Check sheet for the modelled part. Datum: model origin and axes. Units: mm. A direction names the side the tool comes from. Give positions to 0.01 mm unless a question says otherwise; leave off trailing zeros. Order: outer loops, then holes, each group sorted by start corner. A loop starts at its lowest first (then second) coordinate and runs counter-clockwise, first axis right, second up. Notation, with made-up numbers: M 83.25,67.25 L 134.25,67.25 A24 cw 134.25,99.25 Z; hole C 40.25,83.5 d9. An arc over 180 degrees is marked long. Answer in a Markdown table with one row per item. Add a question column.
Autodesk Inventor part; units mm, degrees
ref_plane "YZ Plane" through (0, 0, 0) normal (1, 0, 0) x (0, 1, 0)
ref_plane "XZ Plane" through (0, 0, 0) normal (0, 1, 0) x (-1, 0, 0)
ref_plane "XY Plane" through (0, 0, 0) normal (0, 0, 1) x (1, 0, 0)
sketch "Sketch1" plane through (0, 0, 0) normal (0, 1, 0) x (-1, 0, 0)
  line L0 (0, 0) -> (-120.65, 0)
  line L1 (-120.65, 0) -> (-120.65, -63.5)
  line L2 (-120.65, -63.5) -> (0, -63.5)
  line L3 (0, -63.5) -> (0, 0)
  dimension "d0" = 120.65
  dimension "d1" = 63.5
extrude "Extrusion1" add sketch "Sketch1" along normal blind 3.175
sketch "Sketch2" plane through (0, 0, 0) normal (0, 0, 1) x (1, 0, 0)
  line L0 (0, 0) -> (120.65, 0)
  line L1 (0, 0) -> (120.65, 0)
  line L2 (120.65, 0) -> (120.65, -31.75)
  line L3 (120.65, -31.75) -> (0, -31.75)
  line L4 (0, -31.75) -> (0, 0)
  dimension "d4" = 31.75
extrude "Extrusion2" add sketch "Sketch2" against normal blind 3.175
sketch "Sketch4" plane through (120.65, 0, -63.5) normal (0, 0, -1) x (-1, 0, 0)
  line L0 (0, -31.75) -> (0, 3.175)
  line L1 (120.65, -31.75) -> (120.65, 3.175)
  line L2 (0, 3.175) -> (120.65, 3.175)
  line L3 (120.65, 3.175) -> (120.65, -31.75)
  line L4 (120.65, -31.75) -> (0, -31.75)
  line L5 (0, -31.75) -> (0, 3.175)
  point P0 (120.65, 0)
extrude "Extrusion4" add sketch "Sketch4" against normal blind 3.175
fillet "Fillet1" radius 3.175 1 edges at (60.325, 3.175, 0)
fillet "Fillet2" radius 3.175 1 edges at (60.325, 3.175, -63.5)
sketch "Sketch5" plane through (0, -31.75, 0) normal (0, 0, 1) x (1, 0, 0)
  line L0 (120.65, 0) -> (0, 0)
  line L1 (120.65, 34.925) -> (0, 34.925)
  line L2 (120.65, 0) -> (120.65, 31.75)
  line L3 (0, 0) -> (0, 31.75)
  point P0 (44.069, 17.4625)
  point P1 (76.581, 17.4625)
  point P2 (60.325, 17.4625)
  dimension "d14" = 32.512
  dimension "d15" = 34.925
  dimension "d16" = 17.4625
  dimension "d17" = 17.4625
  dimension "d18" = 120.65
  dimension "d20" = 16.256
  dimension "d21" = 17.4625
  dimension "d22" = 60.325
  dimension "d23" = 16.256
hole "Hole1" at (44.069, -14.2875, 0) at (76.581, -14.2875, 0) direction (0, 0, -1) diameter 3.0625 end through all
properties part number "track bracket"
Q1. Cross-section at B-B (x = 71). Record the boundary of the cut face in (y, z) (3 decimals), and give its area (3 significant figures).
Q2. Cross-section at C-C (z = -5). Record the boundary of the cut face in (x, y) (3 decimals), and give its area (3 significant figures).
Q3. Draft check along Y on faces 1 (the cylindrical face through (42.55, -14.09, -61.93)), 2 (the flat face through (59, -16, -3.175)), 3 (the flat face through (59, -31.75, -62)), 4 (the flat face through (61, 3.175, -31)). Enter one of: pulls with the +Y half, pulls with the -Y half, needs draft (parallel to the pull), parting line crosses it, or undercut.
Q4. Go/stop test with a flat-tipped pin: pin 1 (10 mm diameter, centred on x = 97, z = -38, fed in from -Y). Record where the tip stops, or that it passes through.
Q5. Cross-section at A-A (y = -25.5). Record the boundary of the cut face in (x, z) (3 decimals), and give its area (3 significant figures).
Q6. Tool access check on faces 5 (the flat face through (61, 0, -31)), 6 (the flat face through (59, -16, 0)). Record the directions out of +Z, -Z, +X, -X, +Y, -Y that give a thin tool (end or side, any length) a straight path to the whole face; none if there is none.
Q7. Thickness scan on probe 1 along Z at (x, y) = (96.5, -15) (3 decimals); probe 2 along Y at (x, z) = (111.5, -17.5) (3 decimals); probe 3 along Z at (x, y) = (94, 0.5). Record the ranges inside material, lowest first.
Values follow:
| question | item | result |
|---|---|---|
| 1 | outline | M -31.75,-63.5 L 0,-63.5 A3.175 ccw 3.175,-60.325 L 3.175,-3.175 A3.175 ccw 0,0 L -31.75,0 L -31.75,-3.175 L 0,-3.175 L 0,-60.325 L -31.75,-60.325 Z |
| 1 | area | 399 mm² |
| 2 | outline | M 0,0 L 120.65,0 L 120.65,3.175 L 0,3.175 Z |
| 2 | area | 383 mm² |
| 3 | face 1 | undercut |
| 3 | face 2 | needs draft |
| 3 | face 3 | pulls with the -Y half |
| 3 | face 4 | pulls with the +Y half |
| 4 | pin 1 | y = 0 |
| 5 | outline | M 0,-63.5 L 120.65,-63.5 L 120.65,-60.325 L 0,-60.325 Z; M 0,-3.175 L 120.65,-3.175 L 120.65,0 L 0,0 Z |
| 5 | area | 766 mm² |
| 6 | face 5 | +X, -X, -Y |
| 6 | face 6 | +Z, +X, -X, +Y, -Y |
| 7 | probe 1 | -63.5 to -60.325, -3.175 to 0 |
| 7 | probe 2 | 0 to 3.175 |
| 7 | probe 3 | -63.46 to -0.04 |
